Source: CAD feature listing. Evaluate the final solid. Frame: model axes, mm. Face numbers are marked on the shaded views. Round coordinates to 2 decimals unless told otherwise and drop trailing zeros. Loops run counter-clockwise (first coordinate to the right, second up) from the corner with the lowest first, then second, coordinate; pieces in that order, holes last. Notation, with made-up numbers: (15.5, -10) -> (57.5, -10) arc R19 cw to (57.5, 22) -> close; hole circle Ø11 at (-39.75, -31). An arc over 180 degrees is marked (long way). Return JSON: item names as keys, results as strings. Group by question number.
```python
from build123d import *

# Parameters (mm, degrees)
F0_W     = 15.875
F0_H     = 15.875
F1_DEPTH = 250.825
F4_DEPTH = 317.5
F2_W     = 6.35
F2_H     = 25.4
F2_W_2   = 3.175
F2_H_2   = 19.05
F5_DEPTH = 38.101


with BuildPart() as f1:
    # F0 (on Front) → F1 (new body)
    with BuildSketch(Plane.XZ):
        Polygon((-14.2875, 571.5), (-14.2875, 552.45), (0, 552.45), (0, 533.4), (23.8125, 533.4), (23.8125, 571.5), align=None)
        with Locations((7.9375, 438.15)):
            Rectangle(F0_W, F0_H)
        Polygon((-14.2875, 0), (0, 0), (0, 128.5875), (0, 144.4625), (0, 430.2125), (0, 446.0875), (0, 533.4), (0, 552.45), (-14.2875, 552.45), align=None)
        with Locations((7.9375, 136.525)):
            Rectangle(F0_W, F0_H)
    extrude(amount=F1_DEPTH)

    # F3 (on face) → F4 (cut, through all)
    with BuildSketch(Plane(origin=(0, 0, 128.5875), x_dir=(1, 0, 0), z_dir=(0, 0, -1))):
        with BuildLine():
            Line((0, 250.825), (0, 238.125))
            add(Edge.make_bspline(
                [(0, 238.125), (0.6926233759, 234.4606029013), (1.9236757367, 227.3559423783), (7.1384263146, 219.8390585837), (9.937069342, 216.0543113654), (15.004380788, 207.4287550118), (15.5609760484, 196.837061745), (15.875, 187.325)],
                knots=[0, 0, 0, 0, 0.20885854, 0.3936531927, 0.5285953381, 0.7122340762, 1, 1, 1, 1], degree=3))
            Line((15.875, 187.325), (15.875, 250.825))
            Line((15.875, 250.825), (0, 250.825))
        make_face()
        with BuildLine():
            add(Edge.make_bspline(
                [(0, 12.7), (0.6926233759, 16.3643970987), (1.9236757367, 23.4690576217), (7.1384263146, 30.9859414163), (9.937069342, 34.7706886346), (15.004380788, 43.3962449882), (15.5609760484, 53.987938255), (15.875, 63.5)],
                knots=[0, 0, 0, 0, 0.20885854, 0.3936531927, 0.5285953381, 0.7122340762, 1, 1, 1, 1], degree=3))
            Line((0, 12.7), (0, 0))
            Line((0, 0), (15.875, 0))
            Line((15.875, 0), (15.875, 63.5))
        make_face()
    extrude(amount=-F4_DEPTH, mode=Mode.SUBTRACT)

    # F2 (on face) → F5 (cut, through all)
    with BuildSketch(Plane(origin=(-14.2875, 0, 0), x_dir=(0, -1, 0), z_dir=(-1, 0, 0))):
        with Locations((3.175, 12.7)):
            Rectangle(F2_W, F2_H)
        with Locations((247.65, 12.7)):
            Rectangle(F2_W, F2_H)
        with Locations((249.2375, 561.975)):
            Rectangle(F2_W_2, F2_H_2)
        with Locations((1.5875, 561.975)):
            Rectangle(F2_W_2, F2_H_2)
    extrude(amount=-F5_DEPTH, mode=Mode.SUBTRACT)


solid = f1.part
```
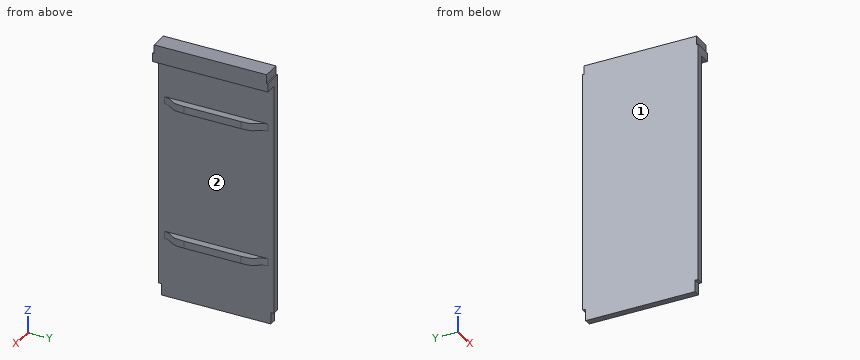
(1) Mould query, pull axis Z, two halves, no side actions, for the marked faces 1 and 2. Classes: released by +Z, released by -Z, zero draft, split by the parting line, or undercut.
(2) Cut plane C-C (z = 326.5). Return loops of the section in (x, y) (1 decimal).
(3) Ray query, line 1 (Z direction, x = 3.5, y = -91); line 2 (X direction, y = -212, z = 234); line 3 (Z direction, x = 20, y = -164.5). Return the intervals inside material, ascending.
(4) Pin query (flat end, axial travel): pin 1 (6 mm diameter, centred on y = -150.5, z = 189.5, fed in from +X); pin 2 (1.9 mm diameter, centred on x = -6, y = -247, fed in from -Z); pin 3 (12 mm diameter, centred on x = 15, y = -104, fed in from -Z). Return the tip coordinate at first contact, or that it passes through.
(5) Cut plane B-B (x = 7). Count the separate pieces of the cut face and the enclosed holes in it, and give its area (3 significant figures).
(6) Cut plane A-A (y = -144). Return loops of the section in (x, z) (1 decimal).
Answers follow:
{
 "1": {"face 1": "zero draft", "face 2": "undercut"},
 "2": {"outline": "(-14.3, -250.8) -> (0, -250.8) -> (0, 0) -> (-14.3, 0) -> close"},
 "3": {"line 1": "128.59 to 144.46, 430.21 to 446.09, 533.4 to 571.5", "line 2": "-14.29 to 0", "line 3": "533.4 to 571.5"},
 "4": {"pin 1": "x = 0", "pin 2": "z = 25.4", "pin 3": "z = 128.59"},
 "5": {"separate pieces": "3", "enclosed holes": "0", "area": "15,400 mm^2"},
 "6": {"outline": "(-14.3, 0) -> (0, 0) -> (0, 128.6) -> (15.9, 128.6) -> (15.9, 144.5) -> (0, 144.5) -> (0, 430.2) -> (15.9, 430.2) -> (15.9, 446.1) -> (0, 446.1) -> (0, 533.4) -> (23.8, 533.4) -> (23.8, 571.5) -> (-14.3, 571.5) -> close"}
}
